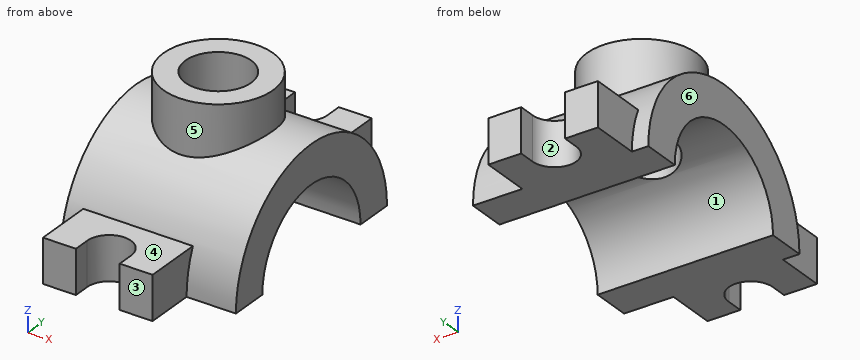
from build123d import *

# Parameters (mm, degrees)
EXTRUDE_1_DEPTH     = 32
SKETCH_2_R          = 10
EXTRUDE_2_DEPTH     = 27
SKETCH_3_W          = 20
SKETCH_3_H          = 58
EXTRUDE_3_DEPTH     = 8
SKETCH_4_R          = 6
CUT_EXTRUDE_1_DEPTH = 51.931326429
CUT_EXTRUDE_2_DEPTH = 51.931326429
CUT_EXTRUDE_4_DEPTH = 8


with BuildPart() as part:
    # 草图1 → 凸台-拉伸1 (new body)
    with BuildSketch(Plane(origin=(0, 0, 0), x_dir=(0, 0, -1), z_dir=(1, 0, 0))):
        with BuildLine():
            Line((0, 20), (0, -20))
            ThreePointArc((0, -20), (-20, 0), (0, 20))
        make_face()
    extrude(amount=EXTRUDE_1_DEPTH)

    # 草图2 → 凸台-拉伸2 (add)
    with BuildSketch(Plane(origin=(0, 0, 0), x_dir=(-1, 0, 0), z_dir=(0, 0, -1))):
        with Locations((-15, 0)):
            Circle(SKETCH_2_R)
    extrude(amount=-EXTRUDE_2_DEPTH)

    # 草图3 → 凸台-拉伸3 (add)
    with BuildSketch(Plane(origin=(0, 0, 0), x_dir=(-1, 0, 0), z_dir=(0, 0, -1))):
        with Locations((-13, 0)):
            Rectangle(SKETCH_3_W, SKETCH_3_H)
    extrude(amount=-EXTRUDE_3_DEPTH)

    # 草图4 → 切除-拉伸1 (cut, through all)
    with BuildSketch(Plane.XY.offset(27)):
        with Locations((15, 0)):
            Circle(SKETCH_4_R)
    extrude(amount=-CUT_EXTRUDE_1_DEPTH, mode=Mode.SUBTRACT)

    # 草图5 → 切除-拉伸2 (cut, through all)
    with BuildSketch(Plane(origin=(32, 0, 0), x_dir=(0, 0, -1), z_dir=(1, 0, 0))):
        with BuildLine():
            Line((0, 13), (0, -13))
            ThreePointArc((0, -13), (-13, 0), (0, 13))
        make_face()
    extrude(amount=-CUT_EXTRUDE_2_DEPTH, mode=Mode.SUBTRACT)

    # 草图6 → 切除-拉伸4 (cut)
    with BuildSketch(Plane(origin=(0, 0, 0), x_dir=(-1, 0, 0), z_dir=(0, 0, -1))):
        with BuildLine():
            Line((-17, 26), (-17, 29))
            Line((-17, 29), (-9, 29))
            Line((-9, 29), (-9, 26))
            ThreePointArc((-9, 26), (-13, 22), (-17, 26))
        make_face()
        with BuildLine():
            Line((-17, -26), (-17, -29))
            Line((-17, -29), (-9, -29))
            Line((-9, -29), (-9, -26))
            ThreePointArc((-9, -26), (-13, -22), (-17, -26))
        make_face()
    extrude(amount=-CUT_EXTRUDE_4_DEPTH, mode=Mode.SUBTRACT)


solid = part.part
Read the model definition and answer for the solid it produces. Units are mm, in the model's axes. Face numbers are marked on the shaded views. A direction names the side the tool comes from. Coordinates: 2 decimals unless noted, no trailing zeros. Write each loop counter-clockwise with the first axis right and the second up, starting at its lowest first coordinate (ties: lowest second). Pieces come first, ordered by that corner, then holes. Notation, with made-up numbers: (55, 61.25) -> (74, 61.25) arc R20 cw to (74, 72.25) -> close; hole circle Ø7 at (87, -3.5). An arc over 180 degrees is marked (long way). Return JSON: item names as keys, results as strings.
(1) The part is cut by section B-B on y = 0. Give the vertices of the cut face in (x, z), then the cut area to 3 significant figures.
Answers below:
{"outline": "(0, 13) -> (9, 13) -> (9, 27) -> (5, 27) -> (5, 20) -> (0, 20) -> close; (21, 13) -> (32, 13) -> (32, 20) -> (25, 20) -> (25, 27) -> (21, 27) -> close", "area": "196 mm^2"}
(2) Consider line 1 along X through (y, z) = (0, 18); line 2 along X through (y, z) = (0, 23.5); line 3 along Y through (x, z) = (15, 17.75). Determine where each line is inside the solid, lowest interval first. Write a range as from..to.
Answers below:
{"line 1": "0..9, 21..32", "line 2": "5..9, 21..25", "line 3": "-10..-6, 6..10"}
(3) The part is cut by section A-A on z = 2.25. Give the vertices of the cut face in (x, y), then the cut area to 3 significant figures.
Answers below:
{"outline": "(0, -19.87) -> (3, -19.87) -> (3, -29) -> (9, -29) -> (9, -26) arc R4 cw to (17, -26) -> (17, -29) -> (23, -29) -> (23, -19.87) -> (32, -19.87) -> (32, -12.8) -> (0, -12.8) -> close; (0, 12.8) -> (32, 12.8) -> (32, 19.87) -> (23, 19.87) -> (23, 29) -> (17, 29) -> (17, 26) arc R4 cw to (9, 26) -> (9, 29) -> (3, 29) -> (3, 19.87) -> (0, 19.87) -> close", "area": "719 mm^2"}
(4) Each of these flat-tipped pins is pushed along its axis until it touches: P1, Ø3.5, axis at y = 28, z = 6, coming from the -X side; P2, Ø8.5, axis at x = 13, y = 21, coming from the +Z side; P3, Ø8, axis at x = 27.5, y = 7, coming from the +Z side. Where does it stop, or does it pass through?
Answers below:
{"P1": "x = 3", "P2": "z = 10.93", "P3": "z = 19.77"}
(5) Which of the six approach directions +Z, -Z, +X, -X, +Y, -Y give full straight-line access (tool end or side, diameter ignored) to the marked faces 4, 5 and 6?
Answers below:
{"face 4": "+Z, +X, -X, -Y", "face 5": "+Z", "face 6": "+Z, -Z, -X, +Y, -Y"}
(6) For a pull along Y with two mould halves and no side action, classify the marked faces 1, 2 and 3 as pulls with the +Y half, pulls with the -Y half, needs draft (parallel to the pull), parting line crosses it, or undercut.
Answers below:
{"face 1": "undercut", "face 2": "pulls with the +Y half", "face 3": "pulls with the -Y half"}
(7) The part is cut by section C-C on x = 12.5. Give the vertices of the cut face in (y, z).
Answers below:
{"outline": "(-22.03, 0) -> (-13, 0) arc R13 cw to (-5.45, 11.8) -> (-5.45, 27) -> (-9.68, 27) -> (-9.68, 17.5) arc R20 ccw to (-18.33, 8) -> (-22.03, 8) -> close; (5.45, 11.8) arc R13 cw to (13, 0) -> (22.03, 0) -> (22.03, 8) -> (18.33, 8) arc R20 ccw to (9.68, 17.5) -> (9.68, 27) -> (5.45, 27) -> close"}
(8) The part is cut by section D-D on z = 24.75. Give the vertices of the cut face in (x, y), then the cut area to 3 significant figures.
Answers below:
{"outline": "circle Ø20 at (15, 0); hole circle Ø12 at (15, 0)", "area": "201 mm^2"}
